Part print with two shaded views. Sizes in mm from the minimum x, y, z corner. Round coordinates to 2 decimals unless told otherwise and drop trailing zeros. Loops run counter-clockwise (first coordinate to the right, second up) from the corner with the lowest first, then second, coordinate; pieces in that order, holes last. Notation, with made-up numbers: M 83,-12.75 L 131,-12.75 A19 ccw 131,1.25 Z; hole C 18,-6.75 d8. An arc over 180 degrees is marked long. Put each result on its own line as item: value. Start each with the question number.
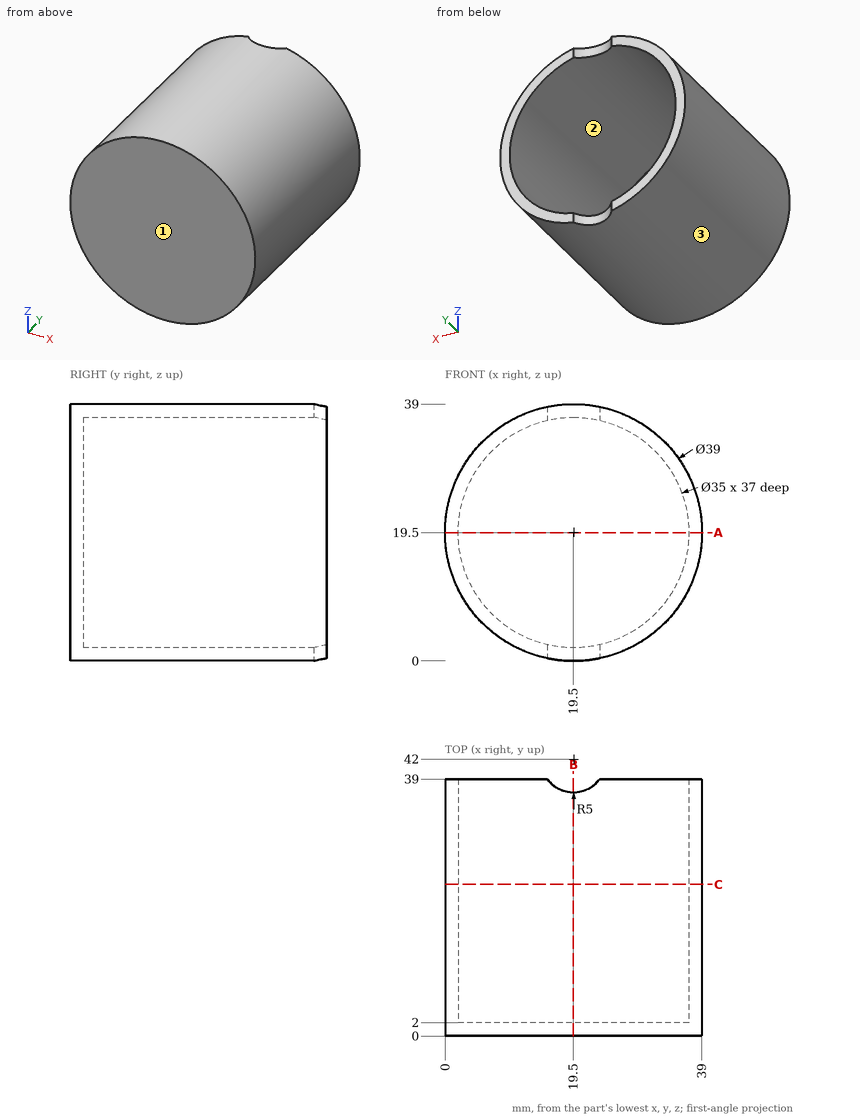
(1) Cut at B-B on x = 19.5. List the corners of the cut face in (y, z).
(2) Cut at C-C on y = 23. List the corners of the cut face in (x, z).
(3) Drill centre lines: line 1 along X through (y, z) = (26, 19); line 2 along Y through (x, z) = (10, 6). Where is each one in solid material? Low to high.
(4) Flat gauge pins, fed straight in: pin 1 Ø10 at (y, z) = (30.5, 9.5) entering from +X; pin 2 Ø1.5 at (x, y) = (15, 9) entering from +Z; pin 3 Ø10 at (x, y) = (32.5, 22) entering from +Z. Where does each tip first touch, or does it go through?
(5) Cut at A-A on z = 19.5. List the corners of the cut face in (x, y), and give its area (3 significant figures).
(6) Mould opens along X. For the marked faces 1, 2 and 3 say: +X half, -X half, draft (parallel to the pull), parting line (faces both ways), or undercut.
Taken from the geometry:
1. outline: M 0,0 L 37,0 L 37,2 L 2,2 L 2,37 L 37,37 L 37,39 L 0,39 Z
2. outline: C 19.5,19.5 d39; hole C 19.5,19.5 d35
3. line 1: 0.01 to 2.01, 36.99 to 38.99
3. line 2: 0 to 2
4. pin 1: x = 38.35
4. pin 2: z = 38.64
4. pin 3: z = 37.28
5. outline: M 0,0 L 39,0 L 39,39 L 37,39 L 37,2 L 2,2 L 2,39 L 0,39 Z
5. area: 226 mm2
6. face 1: draft
6. face 2: undercut
6. face 3: parting line
